```python
from build123d import *

# Parameters (mm, degrees)
SKETCH1_R           = 6.715
SKETCH1_R_2         = 5
BOSS_EXTRUDE1_DEPTH = 17
SKETCH4_R           = 9.4
BOSS_EXTRUDE2_DEPTH = 8
SKETCH7_R           = 11
SKETCH7_R_2         = 9.4
BOSS_EXTRUDE3_DEPTH = 17
SKETCH8_R           = 5
CUT_EXTRUDE1_DEPTH  = 17
FILLET1_R           = 0.5


with BuildPart() as part:
    # Sketch1 → Boss-Extrude1 (new body)
    with BuildSketch(Plane(origin=(0, 0, 0), x_dir=(1, 0, 0), z_dir=(0, 1, 0))):
        with Locations(Location((0, 0, 0), (0, 0, 270))):
            Circle(SKETCH1_R)
        with Locations(Location((0, 0, 0), (0, 0, 270))):
            Circle(SKETCH1_R_2, mode=Mode.SUBTRACT)
    extrude(amount=BOSS_EXTRUDE1_DEPTH)

    # Sketch4 → Boss-Extrude2 (add, symmetric)
    with BuildSketch(Plane(origin=(0, 8.5, 0), x_dir=(1, 0, 0), z_dir=(0, 1, 0))):
        with Locations(Location((0, 0, 0), (0, 0, 270))):
            Circle(SKETCH4_R)
    extrude(amount=BOSS_EXTRUDE2_DEPTH, both=True)

    # Sketch7 → Boss-Extrude3 (add)
    with BuildSketch(Plane(origin=(0, 17, 0), x_dir=(1, 0, 0), z_dir=(0, 1, 0))):
        with Locations(Location((0, 0, 0), (0, 0, 270))):
            Circle(SKETCH7_R)
        with Locations(Location((0, 0, 0), (0, 0, 270))):
            Circle(SKETCH7_R_2, mode=Mode.SUBTRACT)
    extrude(amount=-BOSS_EXTRUDE3_DEPTH)

    # Sketch8 → Cut-Extrude1 (cut)
    with BuildSketch(Plane.XZ.offset(-0.5)):
        with Locations(Location((0, 0, 0), (0, 0, 90))):
            Circle(SKETCH8_R)
    extrude(amount=-CUT_EXTRUDE1_DEPTH, mode=Mode.SUBTRACT)

    # Fillet1
    fillet1_edges = [part.edges().sort_by_distance(p)[0] for p in [
        (0, 0, -11),
        (0, 17, -11),
    ]]
    fillet(fillet1_edges, radius=FILLET1_R)


solid = part.part
```
Model file for the job. Use its own axes, mm. A direction names the side the tool comes from. Coordinates: 2 decimals unless noted, no trailing zeros. Write each loop counter-clockwise with the first axis right and the second up, starting at its lowest first coordinate (ties: lowest second). Pieces come first, ordered by that corner, then holes. Notation, with made-up numbers: (54.25, 45) - (105.25, 45) arc R24 cw to (105.25, 84) - close; hole circle Ø5 at (33, 21). An arc over 180 degrees is marked (long way). One line per item, written item: value. Start each with the question number.
1. Slice it at A-A (z = 0). Write the cut outline in (x, y) (3 decimals).
2. Probe line 1 (X direction, y = 16.7, z = 0) (3 decimals); line 2 (X direction, y = 4.75, z = 0); line 3 (Y direction, x = -6.5, z = 3.5). List the from-to ranges inside material, lowest first. Write a range as from..to.
3. Slice it at B-B (x = 0). Write the cut outline in (y, z) (3 decimals), plus the area to 3 significant figures.
4. Tool access for faces 1 (the cylindrical face through (-2.572, 0.246, 6.203)), 2 (the cylindrical face through (2.824, 16.754, 8.966)), 3 (the flat face through (-9.3, 0, -2.4)): list every direction of +Z, -Z, +X, -X, +Y, -Y with a clear straight run to the whole face (end or side of a thin tool).
5. Slice it at C-C (y = 13). Write the cut outline in (x, z), plus the area to 3 significant figures.
6. Flat gauge pins, fed straight in: pin 1 (10 mm diameter, centred on y = 3.5, z = 6.5, fed in from -X); pin 2 (10 mm diameter, centred on y = 14, z = 7.5, fed in from -X); pin 3 (3 mm diameter, centred on y = 8, z = 2, fed in from +X). Where does each tip first touch, or does it go through?
7. Mould opens along X. For faces 4 (the cylindrical face through (2.824, 0.253, 8.966)), 5 (the flat face through (-9.3, 17, -2.4)), 6 (the cylindrical face through (-10.74, 8.61, -2.38)) say: released by +X, released by -X, zero draft, split by the parting line, or undercut.
Answers below:
1. outline: (-11, 0.5) arc R0.5 ccw to (-10.5, 0) - (-9.4, 0) - (-9.4, 0.5) - (-6.715, 0.5) - (-6.715, 0) - (-5, 0) - (-5, 17) - (-6.715, 17) - (-6.715, 16.5) - (-9.4, 16.5) - (-9.4, 17) - (-10.5, 17) arc R0.5 ccw to (-11, 16.5) - close; (5, 0) - (6.715, 0) - (6.715, 0.5) - (9.4, 0.5) - (9.4, 0) - (10.5, 0) arc R0.5 ccw to (11, 0.5) - (11, 16.5) arc R0.5 ccw to (10.5, 17) - (9.4, 17) - (9.4, 16.5) - (6.715, 16.5) - (6.715, 17) - (5, 17) - close
2. line 1: x = -10.958..-9.4, -6.715..-5, 5..6.715, 9.4..10.958
2. line 2: x = -11..-5, 5..11
2. line 3: y = 0.5..16.5
3. outline: (0, -10.5) arc R0.5 ccw to (0.5, -11) - (16.5, -11) arc R0.5 ccw to (17, -10.5) - (17, -9.4) - (16.5, -9.4) - (16.5, -6.715) - (17, -6.715) - (17, -5) - (0, -5) - (0, -6.715) - (0.5, -6.715) - (0.5, -9.4) - (0, -9.4) - close; (0, 5) - (17, 5) - (17, 6.715) - (16.5, 6.715) - (16.5, 9.4) - (17, 9.4) - (17, 10.5) arc R0.5 ccw to (16.5, 11) - (0.5, 11) arc R0.5 ccw to (0, 10.5) - (0, 9.4) - (0.5, 9.4) - (0.5, 6.715) - (0, 6.715) - close
3. area: 198 mm^2
4. face 1: -Y
4. face 2: +Y
4. face 3: +Z, -Z, +X, -X, -Y
5. outline: circle Ø22 at (0, 0); hole circle Ø10 at (0, 0)
5. area: 302 mm^2
6. pin 1: stops at x = -10.9
6. pin 2: stops at x = -10.71
6. pin 3: stops at x = 10.99
7. face 4: undercut
7. face 5: zero draft
7. face 6: split by the parting line
